Autodesk Inventor part; units mm, degrees
ref_plane "YZ Plane" through (0, 0, 0) normal (1, 0, 0) x (0, 1, 0)
ref_plane "XZ Plane" through (0, 0, 0) normal (0, 1, 0) x (-1, 0, 0)
ref_plane "XY Plane" through (0, 0, 0) normal (0, 0, 1) x (1, 0, 0)
sketch "草圖1" plane through (0, 0, 0) normal (0, 1, 0) x (-1, 0, 0)
  circle A0 centre (0, 0) radius 5.75
  dimension "d0" = 11.5
extrude "擠出1" add sketch "草圖1" along normal blind 2
sketch "草圖2" plane through (0, 0, 0) normal (0, -1, 0) x (1, 0, 0)
  circle A0 centre (0, 0) radius 4.5
  dimension "d3" = 9
extrude "擠出2" add sketch "草圖2" along normal blind 5
sketch "草圖3" plane through (0, -5, 0) normal (0, -1, 0) x (1, 0, 0)
  circle A0 centre (0, 0) radius 5.5
extrude "擠出3" add sketch "草圖3" along normal blind 1
sketch "草圖4" plane through (0, 2, 0) normal (0, 1, 0) x (1, 0, 0)
  line L0 (-1.75, 1.25) -> (1.75, 1.25)
  line L1 (1.75, 1.25) -> (1.75, -1.25)
  line L2 (1.75, -1.25) -> (-1.75, -1.25)
  line L3 (-1.75, -1.25) -> (-1.75, 1.25)
  line L4 (-1.75, 1.25) -> (1.75, -1.25) construction
  line L5 (1.75, 1.25) -> (-1.75, -1.25) construction
  point P0 (0, 0)
  dimension "d8" = 2.5
  dimension "d9" = 3.5
extrude "擠出4" cut sketch "草圖4" against normal through all
sketch "草圖5" plane through (0, 2, 0) normal (0, 1, 0) x (1, 0, 0)
  line L0 (-1.4797, 3) -> (1.5203, 3)
  line L1 (1.5203, 3) -> (1.5203, 6)
  line L2 (1.5203, 6) -> (-1.4797, 6)
  line L3 (-1.4797, 6) -> (-1.4797, 3)
  circle A0 centre (0, 0) radius 4.5
  line L4 (-1.4797, 3) -> (1.5203, 6) construction
  line L5 (1.5203, 3) -> (-1.4797, 6) construction
  point P0 (0.0203, 4.5)
  point P1 (-1.4797, 4.2497)
  point P2 (1.5203, 4.2354)
  dimension "d12" = 3
  dimension "d15" = 3
extrude "擠出5" cut sketch "草圖5" against normal through all contours L3 L2 L1 A0
properties part number "圓形同心線圈內"
The listing builds one solid part. Answer for the finished solid, in the listing's coordinates (mm). A direction names the side the tool comes from. Give positions to 0.01 mm unless a question says otherwise; leave off trailing zeros. Write each loop counter-clockwise with the first axis right and the second up, starting at its lowest first coordinate (ties: lowest second). Pieces come first, ordered by that corner, then holes. Notation, with made-up numbers: (-25, 3) -> (-6, 3) arc R23 ccw to (-6, 23) -> close; hole circle Ø6 at (-20, 48). An arc over 180 degrees is marked (long way). Use one line per item in the form item = value.
1) For a pull along Z with two mould halves and no side action, classify faces 6 (the flat face through (1.75, -2, 0)), 7 (the flat face through (-1.48, 1, -5)), 8 (the cylindrical face through (-0.242, -5.493, 5.495)) as +Z half, -Z half, draft (parallel to the pull), parting line (faces both ways), or undercut.
Result:
face_6 = undercut
face_7 = draft
face_8 = parting line
2) Each of these flat-tipped pins is pushed along its axis until it touches: P1, Ø0.7, axis at y = 1, z = -4.5, coming from the -X side; P2, Ø4, axis at x = 0.5, y = -0.5, coming from the +Z side; P3, Ø1.2, axis at y = -1, z = -0.5, coming from the -X side; P4, Ø1.8, axis at x = -0.5, y = -2.5, coming from the -Z side. Where does it stop, or does it pass through?
Result:
P1 = -3.98
P2 = 5.75
P3 = -4.5
P4 = -4.5
3) A tool of negligible diameter and unlimited length cuts with its end or side. For faces 1 (the flat face through (0, -2, -1.25)), 2 (the flat face through (0, -6, 3)), 3 (the cylindrical face through (-0.59, -1.94, -4.46)), 4 (the flat face through (0.08, 2, 1.43)), 5 (the flat face through (1.52, -5.5, -4.8)), from which of +Z, -Z, +X, -X, +Y, -Y can it reach the whole face along a straight path? Write none if from no direction.
Result:
face_1 = +Y, -Y
face_2 = +Z, -Z, +X, -X, -Y
face_3 = none
face_4 = +Z, -Z, +X, -X, +Y
face_5 = -Z, +Y, -Y
4) Section D-D on x = -3.5 is taken. Write down the section's boundary in (y, z).
Result:
outline = (-6, -4.24) -> (-5, -4.24) -> (-5, -2.83) -> (0, -2.83) -> (0, -4.56) -> (2, -4.56) -> (2, 4.56) -> (0, 4.56) -> (0, 2.83) -> (-5, 2.83) -> (-5, 4.24) -> (-6, 4.24) -> close
5) Straight lines are drawn through the part: probe 1 along Y at (x, z) = (1.75, 4.75); probe 2 along Z at (x, y) = (0.5, -1.25); probe 3 along X at (y, z) = (0.5, -1). For each, find the intervals that lie inside material, in ascending order.
Result:
probe_1 = -6 to -5, 0 to 2
probe_2 = -4.47 to -1.25, 1.25 to 4.47
probe_3 = -5.66 to -1.75, 1.75 to 5.66
6) Section A-A on x = 0 is taken. Write down the section's boundary in (y, z).
Result:
outline = (-6, -4.5) -> (2, -4.5) -> (2, -1.25) -> (-6, -1.25) -> close; (-6, 1.25) -> (2, 1.25) -> (2, 5.75) -> (0, 5.75) -> (0, 4.5) -> (-5, 4.5) -> (-5, 5.5) -> (-6, 5.5) -> close
7) Section B-B on z = 0 is taken. Write down the section's boundary in (x, y).
Result:
outline = (-5.75, 0) -> (-4.5, 0) -> (-4.5, -5) -> (-5.5, -5) -> (-5.5, -6) -> (-1.75, -6) -> (-1.75, 2) -> (-5.75, 2) -> close; (1.75, -6) -> (5.5, -6) -> (5.5, -5) -> (4.5, -5) -> (4.5, 0) -> (5.75, 0) -> (5.75, 2) -> (1.75, 2) -> close
8) Section C-C on y = -5.5 is taken. Write down the section's boundary in (x, z), plus the area to 3 significant figures.
Result:
outline = (-1.48, -5.3) -> (-1.48, -4.25) arc R4.5 ccw to (1.52, -4.24) -> (1.52, -5.29) arc R5.5 ccw (long way) to start; hole (-1.75, -1.25) -> (1.75, -1.25) -> (1.75, 1.25) -> (-1.75, 1.25) -> close
area = 83.2 mm²
